Geometry: see drawing. Coordinates: mm, zero at the bounding-box minimum. Coordinates: 2 decimals unless noted, no trailing zeros. Loops run counter-clockwise (first coordinate to the right, second up) from the corner with the lowest first, then second, coordinate; pieces in that order, holes last.
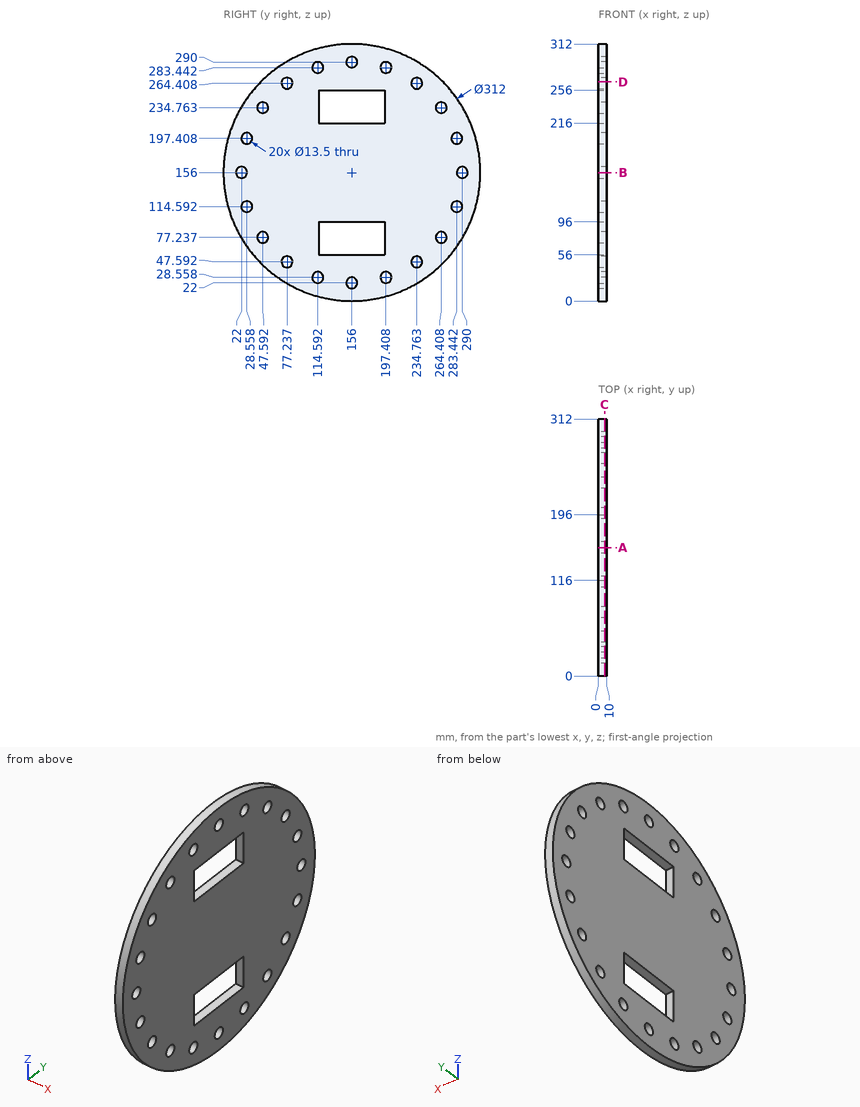
Item 1: Line query: L1, parallel to Y at x = 1, z = 268; L2, parallel to Z at x = 1.5, y = 238 (1 decimal); L3, parallel to Z at x = 4, y = 200 (1 decimal). Output: solid intervals per line, ascending.
Result:
L1: y = 47.41 to 71.52, 82.95 to 229.05, 240.48 to 264.59
L2: z = 23.3 to 41.7, 53.5 to 258.5, 270.3 to 288.7
L3: z = 6.3 to 22.3, 34.8 to 277.2, 289.7 to 305.7
Item 2: Section query D-D (z = 266). Output: boundary loops of the cut face in (x, y), then the cut area to 3 significant figures.
Result:
outline: (0, 45.38) - (10, 45.38) - (10, 70.68) - (0, 70.68) - close; (0, 83.8) - (10, 83.8) - (10, 228.2) - (0, 228.2) - close; (0, 241.32) - (10, 241.32) - (10, 266.62) - (0, 266.62) - close
area: 1,950 mm2
Item 3: Section query C-C (x = 7.5). Count the separate pieces of the cut face and the enclosed holes in it, then the cut area to 3 significant figures.
Result:
separate pieces: 1
enclosed holes: 22
area: 67,200 mm2
Item 4: Section query A-A (y = 156). Output: boundary loops of the cut face in (x, z).
Result:
outline: (0, 0) - (10, 0) - (10, 15.25) - (0, 15.25) - close; (0, 28.75) - (10, 28.75) - (10, 56) - (0, 56) - close; (0, 96) - (10, 96) - (10, 216) - (0, 216) - close; (0, 256) - (10, 256) - (10, 283.25) - (0, 283.25) - close; (0, 296.75) - (10, 296.75) - (10, 312) - (0, 312) - close
Item 5: Contact query for flat-ended pins moving along their axis: P1, Ø11, axis at y = 47.59, z = 77.24, coming from the -X side; P2, Ø5, axis at x = 4, z = 75, coming from the -Y side; P3, Ø1, axis at x = 9, z = 272.5, coming from the +Y side; P4, Ø5, axis at x = 7.5, z = 49, coming from the -Y side (1 decimal). Output: stop coordinate, or through.
Result:
P1: passes through
P2: stops at y = 21.19
P3: stops at y = 260.31
P4: stops at y = 40.2
Item 6: Section query B-B (z = 156). Output: boundary loops of the cut face in (x, y), then the cut area to 3 significant figures.
Result:
outline: (0, 0) - (10, 0) - (10, 15.25) - (0, 15.25) - close; (0, 28.75) - (10, 28.75) - (10, 283.25) - (0, 283.25) - close; (0, 296.75) - (10, 296.75) - (10, 312) - (0, 312) - close
area: 2,850 mm2
